```python
from build123d import *

# Parameters (mm, degrees)
F1_DEPTH      = 2.54
F1_DEPTH_BACK = 2.54
F2_W          = 3.81
F2_H          = 24.638
F2_W_2        = 2.54
F3_DEPTH      = 1.27
F4_W          = 5.715
F4_H          = 2.54
F4_W_2        = 6.35
F6_DEPTH      = 2.54
F5_W          = 6.35
F5_H          = 2.54
F7_DEPTH      = 2.54
F8_T1_DEPTH   = 22.8740361466
F8_T6_DEPTH   = 6.35
F8_T11_DEPTH  = 6.35
F8_T16_DEPTH  = 6.35
F8_T21_DEPTH  = 5.715
F9_W          = 5.842
F9_H          = 1.7639638534
F10_DEPTH     = 1.27
F11_SIZE      = 1.26999


# Not quite as in the source:
# - a fillet or chamfer that OpenCascade refuses, or shapes differently, is made with other operations: its cross-section is extruded or revolved along the edge and cut away or added
# - a fillet or chamfer is up to 0.001 mm smaller than in the source, because OpenCascade refuses the exact size


with BuildPart() as f1:
    # F0 (on Top) → F1 (new body, two sides)
    with BuildSketch(Plane.XY) as f1_sk:
        Polygon((-55.4767026412, 32.9021683285), (-56.7467026412, 32.9021683285), (-56.7467026412, 8.2641683285), (-50.9047026412, 8.2641683285), (-50.9047026412, 32.9021683285), (-52.1747026412, 32.9021683285), (-52.1747026412, 10.0281321819), (-55.4767026412, 10.0281321819), align=None)
    extrude(amount=F1_DEPTH)
    extrude(f1_sk.sketch, amount=-F1_DEPTH_BACK)

    # F2 (on face) → F3 (join)
    with BuildSketch(Plane.XY.offset(2.54)):
        with Locations((-57.3817026412, 20.5831683285)):
            Rectangle(F2_W, F2_H)
        Polygon((-50.9047026412, 8.2641683285), (-55.4767026412, 8.2641683285), (-59.2867026412, 8.2641683285), (-59.2867026412, 5.7241683285), (-48.3647026412, 5.7241683285), (-48.3647026412, 8.2641683285), align=None)
        with Locations((-49.6347026412, 20.5831683285)):
            Rectangle(F2_W_2, F2_H)
        Polygon((-52.1747026412, 10.0281321819), (-55.4767026412, 10.0281321819), (-55.4767026412, 8.2641683285), (-50.9047026412, 8.2641683285), (-50.9047026412, 32.9021683285), (-52.1747026412, 32.9021683285), align=None)
    extrude(amount=F3_DEPTH)

    # F4 (on face) → F6 (join)
    with BuildSketch(Plane(origin=(-56.7467026412, 0, 0), x_dir=(0, -1, 0), z_dir=(-1, 0, 0))):
        with Locations((-30.0446683285, -1.27)):
            Rectangle(F4_W, F4_H)
        with Locations((-11.4391683285, -1.27)):
            Rectangle(F4_W_2, F4_H)
    extrude(amount=F6_DEPTH)

    # F5 (on face) → F7 (join)
    with BuildSketch(Plane.YZ.offset(-50.9047026412)):
        with Locations((29.7271683285, -1.27)):
            Rectangle(F5_W, F5_H)
        with Locations((11.4391683285, -1.27)):
            Rectangle(F5_W, F5_H)
    extrude(amount=F7_DEPTH)

    # F8: chamfer of 2.54 on 6 edges, made by hand

    # F8_s2 → F8_t1 (cut)
    with BuildSketch(Plane.XZ.offset(-32.9021683285)):
        with BuildLine():
            Line((-49.5628605923, -2.611842049), (-52.2465446902, 0.071842049))
            Line((-52.2465446902, 0.071842049), (-52.2973446902, 0.071842049))
            ThreePointArc((-52.2973446902, 0.071842049), (-52.2255026412, -1.2340789755), (-52.2255026412, -2.54))
            Line((-52.2255026412, -2.54), (-52.1747026412, -2.5908))
            ThreePointArc((-52.1747026412, -2.5908), (-50.8687816168, -2.5908), (-49.5628605923, -2.662642049))
            Line((-49.5628605923, -2.662642049), (-49.5628605923, -2.611842049))
        make_face()
        with BuildLine():
            Line((-55.4048605923, 0.071842049), (-58.0885446902, -2.611842049))
            Line((-58.0885446902, -2.611842049), (-58.0885446902, -2.662642049))
            ThreePointArc((-58.0885446902, -2.662642049), (-56.7826236657, -2.5908), (-55.4767026412, -2.5908))
            Line((-55.4767026412, -2.5908), (-55.4259026412, -2.54))
            ThreePointArc((-55.4259026412, -2.54), (-55.4259026412, -1.2340789755), (-55.3540605923, 0.071842049))
            Line((-55.3540605923, 0.071842049), (-55.4048605923, 0.071842049))
        make_face()
    extrude(amount=F8_T1_DEPTH, mode=Mode.SUBTRACT)


with BuildPart() as f8_tool4:
    # F8_s5 → F8_t6 (new body)
    with BuildSketch(Plane.XZ.offset(-32.9021683285)):
        with BuildLine():
            Line((-50.9765446902, 0.071842049), (-48.2928605923, -2.611842049))
            Line((-48.2928605923, -2.611842049), (-48.2420605923, -2.611842049))
            ThreePointArc((-48.2420605923, -2.611842049), (-48.3139026412, -1.3059210245), (-48.3139026412, 0))
            Line((-48.3139026412, 0), (-48.3647026412, 0.0508))
            ThreePointArc((-48.3647026412, 0.0508), (-49.6706236657, 0.0508), (-50.9765446902, 0.122642049))
            Line((-50.9765446902, 0.122642049), (-50.9765446902, 0.071842049))
        make_face()
    extrude(amount=F8_T6_DEPTH)

    split(bisect_by=Plane.YZ.offset(-50.9047026412), keep=Keep.TOP)


with BuildPart() as f1_1:
    add(f1.part)

    # F8_t3: cut F8_tool4
    add(f8_tool4.part, mode=Mode.SUBTRACT)


with BuildPart() as f8_tool9:
    # F8_s10 → F8_t11 (new body)
    with BuildSketch(Plane.XZ.offset(-14.6141683285)):
        with BuildLine():
            Line((-50.9765446902, 0.071842049), (-48.2928605923, -2.611842049))
            Line((-48.2928605923, -2.611842049), (-48.2420605923, -2.611842049))
            ThreePointArc((-48.2420605923, -2.611842049), (-48.3139026412, -1.3059210245), (-48.3139026412, 0))
            Line((-48.3139026412, 0), (-48.3647026412, 0.0508))
            ThreePointArc((-48.3647026412, 0.0508), (-49.6706236657, 0.0508), (-50.9765446902, 0.122642049))
            Line((-50.9765446902, 0.122642049), (-50.9765446902, 0.071842049))
        make_face()
    extrude(amount=F8_T11_DEPTH)

    split(bisect_by=Plane.YZ.offset(-50.9047026412), keep=Keep.TOP)


with BuildPart() as f1_2:
    add(f1_1.part)

    # F8_t8: cut F8_tool9
    add(f8_tool9.part, mode=Mode.SUBTRACT)


with BuildPart() as f8_tool14:
    # F8_s15 → F8_t16 (new body)
    with BuildSketch(Plane.XZ.offset(-8.2641683285)):
        with BuildLine():
            Line((-56.6748605923, 0.071842049), (-59.3585446902, -2.611842049))
            Line((-59.3585446902, -2.611842049), (-59.4093446902, -2.611842049))
            ThreePointArc((-59.4093446902, -2.611842049), (-59.3375026412, -1.3059210245), (-59.3375026412, 0))
            Line((-59.3375026412, 0), (-59.2867026412, 0.0508))
            ThreePointArc((-59.2867026412, 0.0508), (-57.9807816168, 0.0508), (-56.6748605923, 0.122642049))
            Line((-56.6748605923, 0.122642049), (-56.6748605923, 0.071842049))
        make_face()
    extrude(amount=-F8_T16_DEPTH)

    split(bisect_by=Plane.YZ.offset(-56.7467026412), keep=Keep.BOTTOM)


with BuildPart() as f1_3:
    add(f1_2.part)

    # F8_t13: cut F8_tool14
    add(f8_tool14.part, mode=Mode.SUBTRACT)


with BuildPart() as f8_tool19:
    # F8_s20 → F8_t21 (new body)
    with BuildSketch(Plane.XZ.offset(-27.1871683285)):
        with BuildLine():
            Line((-56.6748605923, 0.071842049), (-59.3585446902, -2.611842049))
            Line((-59.3585446902, -2.611842049), (-59.4093446902, -2.611842049))
            ThreePointArc((-59.4093446902, -2.611842049), (-59.3375026412, -1.3059210245), (-59.3375026412, 0))
            Line((-59.3375026412, 0), (-59.2867026412, 0.0508))
            ThreePointArc((-59.2867026412, 0.0508), (-57.9807816168, 0.0508), (-56.6748605923, 0.122642049))
            Line((-56.6748605923, 0.122642049), (-56.6748605923, 0.071842049))
        make_face()
    extrude(amount=-F8_T21_DEPTH)

    split(bisect_by=Plane.YZ.offset(-56.7467026412), keep=Keep.BOTTOM)


with BuildPart() as f1_4:
    add(f1_3.part)

    # F8_t18: cut F8_tool19
    add(f8_tool19.part, mode=Mode.SUBTRACT)

    # F9 (on face) → F10 (cut)
    with BuildSketch(Plane(origin=(0, 0, -2.54), x_dir=(1, 0, 0), z_dir=(0, 0, -1))):
        with Locations((-53.8257026412, -9.1461502552)):
            Rectangle(F9_W, F9_H)
    extrude(amount=-F10_DEPTH, mode=Mode.SUBTRACT)

    # F11 (size 1.27 in the source; OpenCascade refuses exactly that, so slightly less here)
    f11_edges = [f1_4.edges().sort_by_distance(p)[0] for p in [
        (-50.904703, 9.14615, -2.54),
        (-56.746703, 9.14615, -2.54),
    ]]
    chamfer(f11_edges, length=F11_SIZE)


solid = f1_4.part
```
Part model, mm, in its own coordinate system. A direction names the side the tool comes from. Round coordinates to 2 decimals unless told otherwise and drop trailing zeros. Write each loop counter-clockwise with the first axis right and the second up, starting at its lowest first coordinate (ties: lowest second). Pieces come first, ordered by that corner, then holes. Notation, with made-up numbers: (80.25, -2.5) -> (123.25, -2.5) arc R13 cw to (123.25, 2.5) -> close; hole circle Ø2 at (46.25, 9). An arc over 180 degrees is marked (long way). Return JSON: item names as keys, results as strings. Group by question number.
Q1. Mould opens along Y. For faces 5 (the flat face through (-58, 14.614, -2)), 6 (the flat face through (-49.9, 14.614, -1.6)), 7 (the flat face through (-54, 8.264, 0)), 8 (the flat face through (-49.652, 11.484, -1.252)) say: pulls with the +Y half, pulls with the -Y half, needs draft (parallel to the pull), parting line crosses it, or undercut.
Q2. Saw through at A-A on y = 18.5. Write the cut outline in (x, z).
Q3. Saw through at D-D on y = 30.75. Write the cut outline in (x, z).
Q4. Pin check, flat tips, straight feed: pin 1 (1.5 mm diameter, centred on y = 13.5, z = 1, fed in from +X); pin 2 (2 mm diameter, centred on x = -58, z = -1, fed in from -Y); pin 3 (1.4 mm diameter, centred on x = -54, y = 9.5, fed in from -Z). Stop position of each tip, or through.
Q5. Probe L1, parallel to X at y = 25.5, z = 3.25; L2, parallel to X at y = 16, z = 0.5; L3, parallel to Y at x = -57, z = -1. List the from-to ranges inside material, lowest first. Write a range as [from, to].
Q6. Which spindle directions (+Z, -Z, +X, -X, +Y, -Y) get a long thin tool onto all of the face, cutting with end or side? Do faces 1 (the flat face through (-49.9, 26.552, -1.6)), 2 (the flat face through (-52.175, 22, 2)), 3 (the flat face through (-57.999, 30.005, -1.252)), 4 (the flat face through (-58, 27.187, -2)). Say none if no direction does.
Q7. Saw through at C-C on x = -57.25. State how many separate pieces and enclosed holes the cut face has, plus the area to 3 significant figures.
Q8. Saw through at B-B on z = 3.25. Write the cut outline in (x, y).
Answer:
{
 "1": {"face 5": "undercut", "face 6": "undercut", "face 7": "pulls with the -Y half", "face 8": "needs draft"},
 "2": {"outline": "(-59.29, 2.54) -> (-56.75, 2.54) -> (-56.75, -1.27) -> (-55.48, 0) -> (-55.48, 3.81) -> (-59.29, 3.81) -> close; (-52.17, 0) -> (-50.9, -1.27) -> (-50.9, 2.54) -> (-48.36, 2.54) -> (-48.36, 3.81) -> (-52.17, 3.81) -> close"},
 "3": {"outline": "(-59.29, -2.54) -> (-58.02, -2.54) -> (-55.48, 0) -> (-55.48, 3.81) -> (-59.29, 3.81) -> (-59.29, 2.54) -> (-56.75, 2.54) -> (-56.75, 0) -> close; (-52.17, 0) -> (-49.63, -2.54) -> (-48.36, -2.54) -> (-50.9, 0) -> (-50.9, 2.54) -> (-48.36, 2.54) -> (-48.36, 3.81) -> (-52.17, 3.81) -> close"},
 "4": {"pin 1": "x = -50.9", "pin 2": "y = 8.26", "pin 3": "z = -1.27"},
 "5": {"L1": "[-59.29, -55.48], [-52.17, -48.36]", "L2": "[-56.75, -55.48], [-52.17, -50.9]", "L3": "[8.26, 14.61], [27.19, 32.9]"},
 "6": {"face 1": "-Z, +X", "face 2": "+Z, -Z, +Y", "face 3": "-X, +Y, -Y", "face 4": "-Z, -X"},
 "7": {"separate pieces": "3", "enclosed holes": "0", "area": "49.8 mm2"},
 "8": {"outline": "(-59.29, 5.72) -> (-48.36, 5.72) -> (-48.36, 32.9) -> (-52.17, 32.9) -> (-52.17, 10.03) -> (-55.48, 10.03) -> (-55.48, 32.9) -> (-59.29, 32.9) -> close"}
}
